```python
from build123d import *

# Parameters (mm, degrees)
BOSS_EXTRUDE1_DEPTH = 5.334
SKETCH2_W           = 5.334
SKETCH2_H           = 6.1976
SKETCH2_W_2         = 6.1976
SKETCH2_H_2         = 5.334
SKETCH2_W_3         = 7.2136
CUT_EXTRUDE1_DEPTH  = 50.881099186


with BuildPart() as part:
    # Sketch1 → Boss-Extrude1 (new body)
    with BuildSketch(Plane.XY):
        with BuildLine():
            Line((0, 31.75), (0, -5.334))
            Line((0, -5.334), (38.1, -5.334))
            Line((38.1, -5.334), (38.1, 0))
            ThreePointArc((38.1, 0), (29.146926861, 22.105308914), (7.334496124, 31.75))
            Line((7.334496124, 31.75), (5.334, 31.75))
            Line((5.334, 31.75), (0, 31.75))
        make_face()
    extrude(amount=-BOSS_EXTRUDE1_DEPTH)

    # Sketch2 → Cut-Extrude1 (cut, through all)
    with BuildSketch(Plane.XY):
        Polygon((11.684, -5.334), (11.684, 0), (5.334, 0), (5.334, 0.1524), (5.334, 6.35), (0, 6.35), (0, -5.334), align=None)
        with Locations((2.667, 28.6512)):
            Rectangle(SKETCH2_W, SKETCH2_H)
        with Locations((2.667, 15.9512)):
            Rectangle(SKETCH2_W, SKETCH2_H)
        with Locations((21.2852, -2.667)):
            Rectangle(SKETCH2_W_2, SKETCH2_H_2)
        with Locations((34.4932, -2.667)):
            Rectangle(SKETCH2_W_3, SKETCH2_H_2)
    extrude(amount=-CUT_EXTRUDE1_DEPTH, mode=Mode.SUBTRACT)


solid = part.part
```
Read the model definition and answer for the solid it produces. Units are mm, in the model's axes. A direction names the side the tool comes from. Coordinates: 2 decimals unless noted, no trailing zeros. Loops run counter-clockwise (first coordinate to the right, second up) from the corner with the lowest first, then second, coordinate; pieces in that order, holes last.
(1) Flat-ended cylindrical pins translate along their axes: pin 1 Ø2.5 at (x, z) = (2, -2) entering from +Y; pin 2 Ø1.5 at (x, z) = (5.5, -3) entering from -Y; pin 3 Ø1.6 at (y, z) = (-2, -2.5) entering from +X. Find the tip coordinate at first contact, or state that the pin passes through.
Solution:
pin 1: stops at y = 25.55
pin 2: stops at y = 0
pin 3: stops at x = 30.89
(2) The part is cut by section B-B (z = -2.3). Determine the outline of the cut face in (x, y), and give its area (3 significant figures).
Solution:
outline: (0, 6.35) - (5.33, 6.35) - (5.33, 0) - (11.68, 0) - (11.68, -5.33) - (18.19, -5.33) - (18.19, 0) - (24.38, 0) - (24.38, -5.33) - (30.89, -5.33) - (30.89, 0) - (38.1, 0) arc R31.77 ccw to (7.33, 31.75) - (5.33, 31.75) - (5.33, 25.55) - (0, 25.55) - (0, 19.05) - (5.33, 19.05) - (5.33, 12.85) - (0, 12.85) - close
area: 963 mm2
(3) Consider line 1 along Y through (x, z) = (5, -2.5); line 2 along Y through (x, z) = (13.5, -3.2); line 3 along Y through (x, z) = (18, -0.35). Determine where each line is inside the solid, lowest interval first.
Solution:
line 1: y = 6.35 to 12.85, 19.05 to 25.55
line 2: y = -5.33 to 30.95
line 3: y = -5.33 to 29.55
(4) The part is cut by section A-A (x = 4.5). Determine the outline of the cut face in (y, z), and give its area (3 significant figures).
Solution:
outline: (6.35, -5.33) - (12.85, -5.33) - (12.85, 0) - (6.35, 0) - close; (19.05, -5.33) - (25.55, -5.33) - (25.55, 0) - (19.05, 0) - close
area: 69.4 mm2
(5) The part is cut by section C-C (y = 26.5). Determine the outline of the cut face in (x, z).
Solution:
outline: (5.33, -5.33) - (23.85, -5.33) - (23.85, 0) - (5.33, 0) - close
(6) The part is cut by section D-D (x = 26). Determine the outline of the cut face in (y, z).
Solution:
outline: (-5.33, -5.33) - (24.95, -5.33) - (24.95, 0) - (-5.33, 0) - close
(7) A tool of negligible diameter and unlimited length cuts with its end or side. For faces 4 (the face through (18.186, -3, -3)), 5 (the face through (3, 12.852, -3)), 6 (the face through (30.886, -3, -3)), from which of +Z, -Z, +X, -X, +Y, -Y can it reach the whole face along a straight path? Write none if from no direction.
Solution:
face 4: +Z, -Z, -Y
face 5: +Z, -Z, -X
face 6: +Z, -Z, +X, -Y
(8) The mould has two halves that part along Y. Classify faces 1 (the face through (11.684, -3, -3)), 2 (the face through (5.334, 16, -3)), 3 (the face through (3, 25.552, -3)): released by +Y, released by -Y, zero draft, split by the parting line, or undercut.
Solution:
face 1: zero draft
face 2: undercut
face 3: released by +Y
